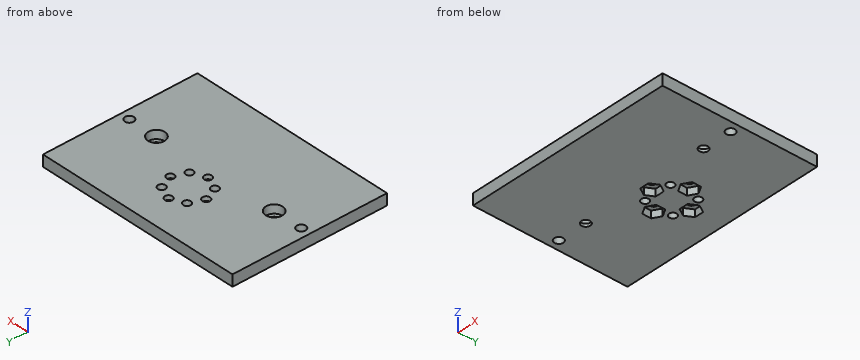
```python
from build123d import *

# Parameters (mm, degrees)
SKETCH_1_W          = 74
SKETCH_1_H          = 55
EXTRUDE_1_DEPTH     = 4
SKETCH_2_R          = 1.6
CUT_EXTRUDE_1_DEPTH = 5
SKETCH_2_3_R        = 1.35
CUT_EXTRUDE_2_DEPTH = 5
CUT_EXTRUDE_3_DEPTH = 2.5
SKETCH_5_R          = 3
CUT_EXTRUDE_4_DEPTH = 3


with BuildPart() as part:
    # 草圖1 → 填料-伸長1 (new body)
    with BuildSketch(Plane.XY):
        Rectangle(SKETCH_1_W, SKETCH_1_H)
    extrude(amount=EXTRUDE_1_DEPTH)

    # 草圖2 → 除料-伸長1 (cut, through all)
    with BuildSketch(Plane.XY.offset(4)):
        with Locations((-33.55, -0.1)):
            Circle(SKETCH_2_R)
        with Locations((33.55, -0.1)):
            Circle(SKETCH_2_R)
        with Locations((-23, -0.1)):
            Circle(SKETCH_2_R)
        with Locations((23, -0.1)):
            Circle(SKETCH_2_R)
    extrude(amount=-CUT_EXTRUDE_1_DEPTH, mode=Mode.SUBTRACT)

    # 草圖2<3> → 除料-伸長2 (cut, through all)
    with BuildSketch(Plane.XY.offset(4)):
        with Locations((0, 2.5)):
            Circle(SKETCH_2_3_R)
        with Locations((4.949747468, 4.550252532)):
            Circle(SKETCH_2_3_R)
        with Locations((7, 9.5)):
            Circle(SKETCH_2_3_R)
        with Locations((4.949747468, 14.449747468)):
            Circle(SKETCH_2_3_R)
        with Locations((-4.949747468, 14.449747468)):
            Circle(SKETCH_2_3_R)
        with Locations((-7, 9.5)):
            Circle(SKETCH_2_3_R)
        with Locations((-4.949747468, 4.550252532)):
            Circle(SKETCH_2_3_R)
        with Locations((0, 16.5)):
            Circle(SKETCH_2_3_R)
    extrude(amount=-CUT_EXTRUDE_2_DEPTH, mode=Mode.SUBTRACT)

    # 草圖3 → 除料-伸長3 (cut)
    with BuildSketch(Plane(origin=(0, 0, 0), x_dir=(-1, 0, 0), z_dir=(0, 0, -1))):
        Polygon((-1.58771324, 19.25), (1.58771324, 19.25), (3.175426481, 16.5), (1.58771324, 13.75), (-1.58771324, 13.75), (-3.175426481, 16.5), align=None)
        Polygon((9.75, 7.91228676), (7, 6.324573519), (4.25, 7.91228676), (4.25, 11.08771324), (7, 12.675426481), (9.75, 11.08771324), align=None)
        Polygon((-1.58771324, -0.25), (-3.175426481, 2.5), (-1.58771324, 5.25), (1.58771324, 5.25), (3.175426481, 2.5), (1.58771324, -0.25), align=None)
        Polygon((-9.75, 11.08771324), (-7, 12.675426481), (-4.25, 11.08771324), (-4.25, 7.91228676), (-7, 6.324573519), (-9.75, 7.91228676), align=None)
    extrude(amount=-CUT_EXTRUDE_3_DEPTH, mode=Mode.SUBTRACT)

    # 草圖5 → 除料-伸長4 (cut)
    with BuildSketch(Plane.XY.offset(4)):
        with Locations((23, -0.1)):
            Circle(SKETCH_5_R)
        with Locations((-23, -0.1)):
            Circle(SKETCH_5_R)
    extrude(amount=-CUT_EXTRUDE_4_DEPTH, mode=Mode.SUBTRACT)


solid = part.part
```
Could you check a few things on this model? Use its own coordinates, in mm. Coordinates: 2 decimals unless noted, no trailing zeros. Order: outer loops, then holes, each group sorted by start corner. A loop starts at its lowest first (then second) coordinate and runs counter-clockwise, first axis right, second up. Notation, with made-up numbers: M -22.5,47.5 L -5.5,47.5 A25 ccw -5.5,80.5 Z; hole C 4,68.25 d6. An arc over 180 degrees is marked long. Use a Markdown table: item, result. Add a question column.
Q1. I want a section at A-A on x = 0. List the corners of the cut face in (y, z) for me, then the cut area to 3 significant figures.
Q2. I want a section at B-B on x = -33.55. List the corners of the cut face in (y, z) for me.
Q3. If I drill on L1, parallel to X at y = 9.5, z = 2; L2, parallel to X at y = 0, z = 2.65; L3, parallel to Y at x = 0, z = 3.25, over which ranges is the centre line in solid material (lowest first)?
Q4. I'm going to push flat-ended pins straight in: pin 1 (6 mm diameter, centred on x = -7.5, y = 10, fed in from -Z); pin 2 (1.6 mm diameter, centred on x = -4.95, y = 4.55, fed in from +Z). Where does each tip first touch, or does it pass through?
Checked values:
| question | item | result |
|---|---|---|
| 1 | outline | M -27.5,0 L -0.25,0 L -0.25,2.5 L 1.15,2.5 L 1.15,4 L -27.5,4 Z; M 3.85,2.5 L 5.25,2.5 L 5.25,0 L 13.75,0 L 13.75,2.5 L 15.15,2.5 L 15.15,4 L 3.85,4 Z; M 17.85,2.5 L 19.25,2.5 L 19.25,0 L 27.5,0 L 27.5,4 L 17.85,4 Z |
| 1 | area | 184 mm² |
| 2 | outline | M -27.5,0 L -1.7,0 L -1.7,4 L -27.5,4 Z; M 1.5,0 L 27.5,0 L 27.5,4 L 1.5,4 Z |
| 3 | L1 | -37 to -9.75, -4.25 to 4.25, 9.75 to 37 |
| 3 | L2 | -37 to -35.15, -31.95 to -26, -20 to 20, 26 to 31.95, 35.15 to 37 |
| 3 | L3 | -27.5 to 1.15, 3.85 to 15.15, 17.85 to 27.5 |
| 4 | pin 1 | z = 0 |
| 4 | pin 2 | through |
